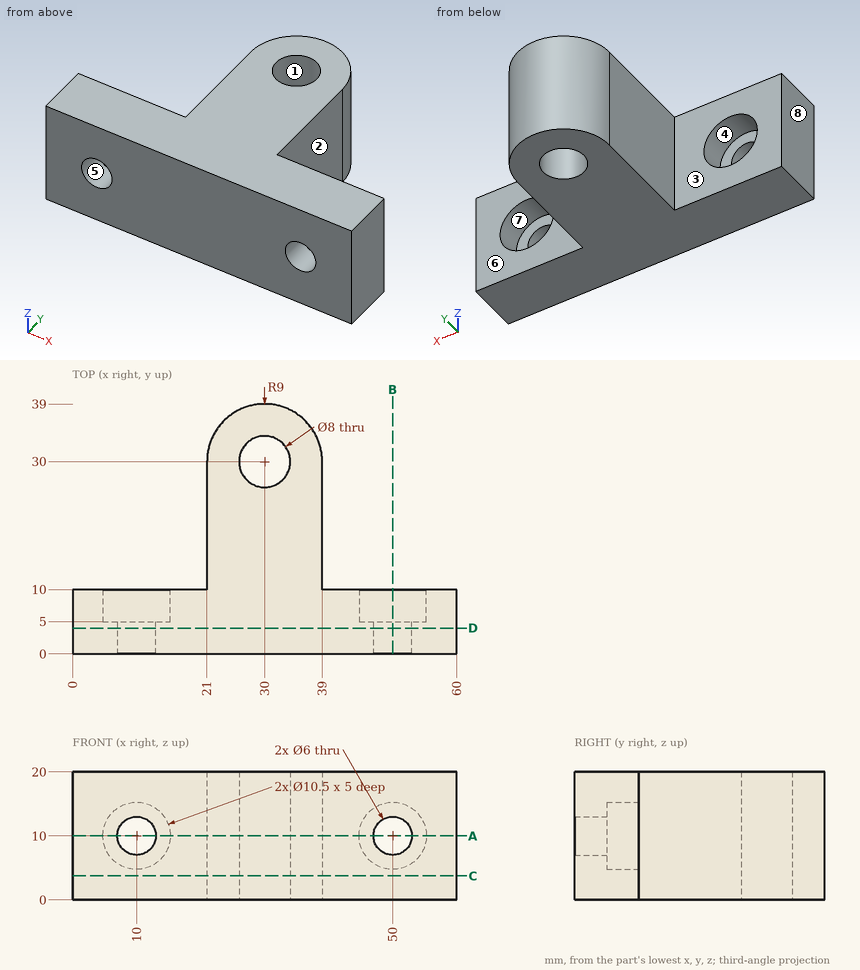
Check sheet for the drawn part. Datum: minimum x, y, z corner. Units: mm. A direction names the side the tool comes from. Give positions to 0.01 mm unless a question says otherwise; leave off trailing zeros. Order: outer loops, then holes, each group sorted by start corner. A loop starts at its lowest first (then second) coordinate and runs counter-clockwise, first axis right, second up. Notation, with made-up numbers: (42, 33.5) -> (46, 33.5) arc R17 ccw to (46, 64.5) -> close; hole circle Ø9 at (10, 30). An arc over 180 degrees is marked (long way). Use a Markdown table: item, result.
1) Tool access check on the marked faces 1, 2, 3 and 4. Record the directions out of +Z, -Z, +X, -X, +Y, -Y that give a thin tool (end or side, any length) a straight path to the whole face; none if there is none.
Results:
| item | result |
|---|---|
| face 1 | +Z, -Z |
| face 2 | +Z, -Z, +X, +Y |
| face 3 | +Z, -Z, -X, +Y |
| face 4 | +Y |
2) Section check D-D, the plane y = 4. Record the boundary of the cut face in (x, z), then the cut area to 3 significant figures.
Results:
| item | result |
|---|---|
| outline | (0, 0) -> (60, 0) -> (60, 20) -> (0, 20) -> close; hole circle Ø6 at (10, 10); hole circle Ø6 at (50, 10) |
| area | 1,140 mm² |
3) Depth check by flat-ended pin: pin 1 Ø1 at (y, z) = (22, 3) entering from +X; pin 2 Ø1 at (x, y) = (32, 30) entering from -Z; pin 3 Ø5 at (y, z) = (22.5, 6) entering from -X; pin 4 Ø6 at (x, z) = (45.5, 13) entering from +Y. Enter the tip coordinate at first touch or a pass-through.
Results:
| item | result |
|---|---|
| pin 1 | x = 39 |
| pin 2 | through |
| pin 3 | x = 21 |
| pin 4 | y = 10 |
4) Section check A-A, the plane z = 10. Record the boundary of the cut face in (x, y), then the cut area to 3 significant figures.
Results:
| item | result |
|---|---|
| outline | (0, 0) -> (7, 0) -> (7, 5) -> (4.75, 5) -> (4.75, 10) -> (0, 10) -> close; (13, 0) -> (47, 0) -> (47, 5) -> (44.75, 5) -> (44.75, 10) -> (39, 10) -> (39, 30) arc R9 ccw to (21, 30) -> (21, 10) -> (15.25, 10) -> (15.25, 5) -> (13, 5) -> close; (53, 0) -> (60, 0) -> (60, 10) -> (55.25, 10) -> (55.25, 5) -> (53, 5) -> close; hole circle Ø8 at (30, 30) |
| area | 872 mm² |
5) Section check C-C, the plane z = 3.75. Record the boundary of the cut face in (x, y), then the cut area to 3 significant figures.
Results:
| item | result |
|---|---|
| outline | (0, 0) -> (60, 0) -> (60, 10) -> (39, 10) -> (39, 30) arc R9 ccw to (21, 30) -> (21, 10) -> (0, 10) -> close; hole circle Ø8 at (30, 30) |
| area | 1,040 mm² |
6) Material ranges on probe 1 along Z at (x, y) = (50, 2.5); probe 2 along Z at (x, y) = (10, 7.85); probe 3 along Y at (x, z) = (30, 17.5), recorded low to high.
Results:
| item | result |
|---|---|
| probe 1 | 0 to 7, 13 to 20 |
| probe 2 | 0 to 4.75, 15.25 to 20 |
| probe 3 | 0 to 26, 34 to 39 |
7) Mould release check, pull along X, two halves, no side actions. Record for the marked faces 5, 6, 7 and 8: pulls with the +X half, pulls with the -X half, needs draft (parallel to the pull), parting line crosses it, or undercut.
Results:
| item | result |
|---|---|
| face 5 | undercut |
| face 6 | needs draft |
| face 7 | undercut |
| face 8 | pulls with the -X half |
8) Section check B-B, the plane x = 50. Record the boundary of the cut face in (y, z), then the cut area to 4 significant figures.
Results:
| item | result |
|---|---|
| outline | (0, 0) -> (10, 0) -> (10, 4.75) -> (5, 4.75) -> (5, 7) -> (0, 7) -> close; (0, 13) -> (5, 13) -> (5, 15.25) -> (10, 15.25) -> (10, 20) -> (0, 20) -> close |
| area | 117.5 mm² |
